Design review of the part built by this model. Coordinates are the model's own, in mm. Give positions to 0.01 mm unless a question says otherwise; leave off trailing zeros. Write each loop counter-clockwise with the first axis right and the second up, starting at its lowest first coordinate (ties: lowest second). Pieces come first, ordered by that corner, then holes. Notation, with made-up numbers: (8.5, -15.5) -> (28.5, -15.5) arc R20 cw to (28.5, 7.5) -> close; hole circle Ø6 at (72.25, 84.25). An arc over 180 degrees is marked (long way). Use CSV: the item, a comma, the result in double quotes.
```python
from build123d import *

# Parameters (mm, degrees)
SKETCH3_R              = 100
SKETCH3_R_2            = 80
BOSS_EXTRUDE1_DEPTH    = 3
SPLIT2_SURFACE_1_BACK  = 283.859
SPLIT2_SURFACE_1_DEPTH = 567.718
SPLIT2_SURFACE_2_BACK  = 283.859
SPLIT2_SURFACE_2_DEPTH = 567.718
BODY_DELETE1_DEPTH     = 3
SKETCH5_R              = 15
BOSS_EXTRUDE2_DEPTH    = 3
SKETCH6_R              = 3.21
CUT_EXTRUDE1_DEPTH     = 3
SPLIT3_SURFACE_3_BACK  = 209.781
SPLIT3_SURFACE_3_DEPTH = 419.562
SPLIT3_SURFACE_4_BACK  = 209.781
SPLIT3_SURFACE_4_DEPTH = 419.562
SPLIT4_SURFACE_5_BACK  = 209.781
SPLIT4_SURFACE_5_DEPTH = 419.562
SPLIT4_SURFACE_6_BACK  = 209.781
SPLIT4_SURFACE_6_DEPTH = 419.562
FILLET1_R              = 10
SPLIT5_SURFACE_7_BACK  = 207.768
SPLIT5_SURFACE_7_DEPTH = 415.536
SPLIT5_SURFACE_8_BACK  = 207.768
SPLIT5_SURFACE_8_DEPTH = 415.536


# Read off the part's stored shape, not the designer's step: Body-Delete1
with BuildPart() as part:
    # Sketch3 → Boss-Extrude1 (new body)
    with BuildSketch(Plane(origin=(0, 0, 0), x_dir=(1, 0, 0), z_dir=(0, 1, 0))):
        with Locations(Location((0, 0, 0), (0, 0, 270))):
            Circle(SKETCH3_R)
        with Locations(Location((0, 0, 0), (0, 0, 270))):
            Circle(SKETCH3_R_2, mode=Mode.SUBTRACT)
    extrude(amount=BOSS_EXTRUDE1_DEPTH)


with BuildPart() as body_2:
    # Split2: the piece behind the surface
    add(part.part)
    # Split2 surface: a surface, the sketch's curves swept straight by 567.718 mm
    with BuildLine(Plane(origin=(0, 3, 0), x_dir=(1, 0, 0), z_dir=(0, 1, 0)).offset(-SPLIT2_SURFACE_1_BACK), mode=Mode.PRIVATE) as split2_surface_1_path:
        Line((69.282032303, 72.111025509), (69.282032303, 40))
        Line((69.282032303, 40), (69.282032303, 0))
        Line((69.282032303, 0), (-114.167790304, 0))
        Line((-114.167790304, 0), (-114.167790304, -108.297460661))
        Line((-114.167790304, -108.297460661), (110.524137422, -108.297460661))
        Line((110.524137422, -108.297460661), (110.524137422, 72.111025509))
        Line((110.524137422, 72.111025509), (69.282032303, 72.111025509))
    split2_surface_1 = Shell.extrude(split2_surface_1_path.wire(), (0 * SPLIT2_SURFACE_1_DEPTH, 1 * SPLIT2_SURFACE_1_DEPTH, 0 * SPLIT2_SURFACE_1_DEPTH))
    split(bisect_by=split2_surface_1, keep=Keep.BOTTOM)

    # Sketch5 → Boss-Extrude2 (add)
    with BuildSketch(Plane(origin=(0, 3, 0), x_dir=(1, 0, 0), z_dir=(0, 1, 0))):
        with Locations((-89.945938306, 0)):
            Circle(SKETCH5_R)
    extrude(amount=-BOSS_EXTRUDE2_DEPTH)

    # Sketch6 → Cut-Extrude1 (cut)
    with BuildSketch(Plane(origin=(0, 3, 0), x_dir=(1, 0, 0), z_dir=(0, 1, 0))):
        with Locations(Location((-89.945938306, 0, 0), (0, 0, 270))):
            Circle(SKETCH6_R)
    extrude(amount=-CUT_EXTRUDE1_DEPTH, mode=Mode.SUBTRACT)


with BuildPart() as part_1:
    add(part.part)

    # Split2: split by a surface, the side it looks to stays
    # Split2 surface: a surface, the sketch's curves swept straight by 567.718 mm
    with BuildLine(Plane(origin=(0, 3, 0), x_dir=(1, 0, 0), z_dir=(0, 1, 0)).offset(-SPLIT2_SURFACE_2_BACK), mode=Mode.PRIVATE) as split2_surface_2_path:
        Line((69.282032303, 72.111025509), (69.282032303, 40))
        Line((69.282032303, 40), (69.282032303, 0))
        Line((69.282032303, 0), (-114.167790304, 0))
        Line((-114.167790304, 0), (-114.167790304, -108.297460661))
        Line((-114.167790304, -108.297460661), (110.524137422, -108.297460661))
        Line((110.524137422, -108.297460661), (110.524137422, 72.111025509))
        Line((110.524137422, 72.111025509), (69.282032303, 72.111025509))
    split2_surface_2 = Shell.extrude(split2_surface_2_path.wire(), (0 * SPLIT2_SURFACE_2_DEPTH, 1 * SPLIT2_SURFACE_2_DEPTH, 0 * SPLIT2_SURFACE_2_DEPTH))
    split(bisect_by=split2_surface_2, keep=Keep.TOP)

    # Body-Delete1 outline → Body-Delete1 (cut)
    with BuildSketch(Plane(origin=(0, 0, 0), x_dir=(1, 0, 0), z_dir=(0, 1, 0))):
        with BuildLine():
            ThreePointArc((-100, 0), (39.190539482, -92.000552255), (69.282032303, 72.111025509))
            Line((69.282032303, 72.111025509), (69.282032303, 40))
            ThreePointArc((69.282032303, 40), (20.705523608, -77.274066103), (-80, 0))
            Line((-80, 0), (-100, 0))
        make_face()
    extrude(amount=BODY_DELETE1_DEPTH, mode=Mode.SUBTRACT)


with BuildPart() as body_2_2:
    # Split3: the piece behind the surface
    add(body_2.part)
    # Split3 surface: a surface, the sketch's curves swept straight by 419.562 mm
    with BuildLine(Plane(origin=(0, 3, 0), x_dir=(1, 0, 0), z_dir=(0, 1, 0)).offset(-SPLIT3_SURFACE_3_BACK), mode=Mode.PRIVATE) as split3_surface_3_path:
        Line((69.282032303, 40), (59.018656665, 80.726688062))
        Line((59.018656665, 80.726688062), (73.479070656, 80.726688062))
        Line((73.479070656, 80.726688062), (69.282032303, 40))
    split3_surface_3 = Shell.extrude(split3_surface_3_path.wire(), (0 * SPLIT3_SURFACE_3_DEPTH, 1 * SPLIT3_SURFACE_3_DEPTH, 0 * SPLIT3_SURFACE_3_DEPTH))
    split(bisect_by=split3_surface_3, keep=Keep.BOTTOM)


with BuildPart() as body_2_1:
    add(body_2.part)

    # Split3: split by a surface, the side it looks to stays
    # Split3 surface: a surface, the sketch's curves swept straight by 419.562 mm
    with BuildLine(Plane(origin=(0, 3, 0), x_dir=(1, 0, 0), z_dir=(0, 1, 0)).offset(-SPLIT3_SURFACE_4_BACK), mode=Mode.PRIVATE) as split3_surface_4_path:
        Line((69.282032303, 40), (59.018656665, 80.726688062))
        Line((59.018656665, 80.726688062), (73.479070656, 80.726688062))
        Line((73.479070656, 80.726688062), (69.282032303, 40))
    split3_surface_4 = Shell.extrude(split3_surface_4_path.wire(), (0 * SPLIT3_SURFACE_4_DEPTH, 1 * SPLIT3_SURFACE_4_DEPTH, 0 * SPLIT3_SURFACE_4_DEPTH))
    split(bisect_by=split3_surface_4, keep=Keep.TOP)


with BuildPart() as body_2_3:
    # Split4: the piece behind the surface
    add(body_2_1.part)
    # Split4 surface: a surface, the sketch's curves swept straight by 419.562 mm
    with BuildLine(Plane(origin=(0, 3, 0), x_dir=(1, 0, 0), z_dir=(0, 1, 0)).offset(-SPLIT4_SURFACE_5_BACK), mode=Mode.PRIVATE) as split4_surface_5_path:
        Line((66.865251706, 49.590165356), (62.98651951, 48.612701009))
        Line((62.98651951, 48.612701009), (66.652010809, 34.067455273))
        Line((66.652010809, 34.067455273), (71.500426054, 35.289285706))
        Line((71.500426054, 35.289285706), (67.834934755, 49.834531442))
        Line((67.834934755, 49.834531442), (66.865251706, 49.590165356))
    split4_surface_5 = Shell.extrude(split4_surface_5_path.wire(), (0 * SPLIT4_SURFACE_5_DEPTH, 1 * SPLIT4_SURFACE_5_DEPTH, 0 * SPLIT4_SURFACE_5_DEPTH))
    split(bisect_by=split4_surface_5, keep=Keep.BOTTOM)

    # Fillet1
    # the kernel refuses this fillet: 10 mm, written as the material it takes off along each edge
    with BuildSketch(Plane(origin=(63.446918188, 16.684080126, -48.728724305), x_dir=(-0.6358841650465459, 0, -0.7717845092012777), z_dir=(0, -1, 0))) as fillet1_piece_1:
        with BuildLine():
            CenterArc((5.815734054, 9.994146598), FILLET1_R, 222.907386502, 45.132130872)
            Line((-1.508817296, 3.185993579), (-1.655308323, 3.049830519))
            ThreePointArc((-1.655308323, 3.049830519), (-0.935163624, 1.507395163), (-0.180754976, -0.085601627))
            Line((-0.180754976, -0.085601627), (0.00684204, -0.199882932))
            ThreePointArc((0.00684204, -0.199882932), (2.736816025, -0.153172783), (5.46679001, -0.199882932))
            Line((5.46679001, -0.199882932), (5.47363205, 0))
        make_face()
    extrude(amount=30.368160252, mode=Mode.SUBTRACT)


with BuildPart() as body_2_4:
    add(body_2_1.part)

    # Split4: split by a surface, the side it looks to stays
    # Split4 surface: a surface, the sketch's curves swept straight by 419.562 mm
    with BuildLine(Plane(origin=(0, 3, 0), x_dir=(1, 0, 0), z_dir=(0, 1, 0)).offset(-SPLIT4_SURFACE_6_BACK), mode=Mode.PRIVATE) as split4_surface_6_path:
        Line((66.865251706, 49.590165356), (62.98651951, 48.612701009))
        Line((62.98651951, 48.612701009), (66.652010809, 34.067455273))
        Line((66.652010809, 34.067455273), (71.500426054, 35.289285706))
        Line((71.500426054, 35.289285706), (67.834934755, 49.834531442))
        Line((67.834934755, 49.834531442), (66.865251706, 49.590165356))
    split4_surface_6 = Shell.extrude(split4_surface_6_path.wire(), (0 * SPLIT4_SURFACE_6_DEPTH, 1 * SPLIT4_SURFACE_6_DEPTH, 0 * SPLIT4_SURFACE_6_DEPTH))
    split(bisect_by=split4_surface_6, keep=Keep.TOP)


with BuildPart() as body_2_4_1:
    # Split5: the piece behind the surface
    add(body_2_3.part)
    # Split5 surface: a surface, the sketch's curves swept straight by 415.536 mm
    with BuildLine(Plane(origin=(0, 3, 0), x_dir=(1, 0, 0), z_dir=(0, 1, 0)).offset(-SPLIT5_SURFACE_7_BACK), mode=Mode.PRIVATE) as split5_surface_7_path:
        Line((60.973585358, 72.969223669), (58.06453621, 72.23612541))
        Line((58.06453621, 72.23612541), (60.508197077, 62.539294919))
        Line((60.508197077, 62.539294919), (68.981543377, 64.674630251))
        Line((68.981543377, 64.674630251), (66.537882511, 74.371460742))
        Line((66.537882511, 74.371460742), (60.973585358, 72.969223669))
    split5_surface_7 = Shell.extrude(split5_surface_7_path.wire(), (0 * SPLIT5_SURFACE_7_DEPTH, 1 * SPLIT5_SURFACE_7_DEPTH, 0 * SPLIT5_SURFACE_7_DEPTH))
    split(bisect_by=split5_surface_7, keep=Keep.BOTTOM)


with BuildPart() as body_2_3_1:
    add(body_2_3.part)

    # Split5: split by a surface, the side it looks to stays
    # Split5 surface: a surface, the sketch's curves swept straight by 415.536 mm
    with BuildLine(Plane(origin=(0, 3, 0), x_dir=(1, 0, 0), z_dir=(0, 1, 0)).offset(-SPLIT5_SURFACE_8_BACK), mode=Mode.PRIVATE) as split5_surface_8_path:
        Line((60.973585358, 72.969223669), (58.06453621, 72.23612541))
        Line((58.06453621, 72.23612541), (60.508197077, 62.539294919))
        Line((60.508197077, 62.539294919), (68.981543377, 64.674630251))
        Line((68.981543377, 64.674630251), (66.537882511, 74.371460742))
        Line((66.537882511, 74.371460742), (60.973585358, 72.969223669))
    split5_surface_8 = Shell.extrude(split5_surface_8_path.wire(), (0 * SPLIT5_SURFACE_8_DEPTH, 1 * SPLIT5_SURFACE_8_DEPTH, 0 * SPLIT5_SURFACE_8_DEPTH))
    split(bisect_by=split5_surface_8, keep=Keep.TOP)


solid = body_2_4_1.part
```
(1) For line 1 along X through (y, z) = (2.25, 0); line 2 along X through (y, z) = (2.65, -44.5); line 3 along X through (y, z) = (0.5, -63.5), list the stretches that pass through material, from the lowest coordinate up. Write a range as [from, to].
Established:
line 1,"x = [-104.95, -93.16], [-86.74, -74.95]"
line 2,"x = [-89.55, -66.48]"
line 3,"x = [-77.25, -48.66], [48.66, 60.27]"
(2) Mouldability with a two-part tool opening along Z and no side actions: class faces 1 (the face through (-45, 3, -68)), 2 (the face through (63.13, 1.52, -50.56)), 3 (the face through (-38.614, 1.479, -92.244)), 4 (the face through (-92.794, 1.521, 1.481)) as +Z half, -Z half, draft (parallel to the pull), parting line (faces both ways), or undercut.
Established:
face 1,"draft"
face 2,"+Z half"
face 3,"-Z half"
face 4,"undercut"
(3) Take a section at A-A (z = 0). Write out the cut boundary in (x, y).
Established:
outline,"(-104.95, 0) -> (-93.16, 0) -> (-93.16, 3) -> (-104.95, 3) -> close; (-86.74, 0) -> (-74.95, 0) -> (-74.95, 3) -> (-86.74, 3) -> close"
(4) Take a section at C-C (x = -71). Write out the cut boundary in (y, z), then the cut area to 3 significant figures.
Established:
outline,"(0, -70.42) -> (3, -70.42) -> (3, -36.86) -> (0, -36.86) -> close"
area,"101 mm2"
(5) Clearance check with flat-ended pins moving along their axes: pin 1 (1 mm diameter, centred on y = 2.5, z = 2.5, fed in from -X); pin 2 (6 mm diameter, centred on x = -89.95, z = 0, fed in from -Y); pin 3 (1.5 mm diameter, centred on x = 18.5, y = 2, fed in from +Z). State where each tip first meets the part, or that it passes through.
Established:
pin 1,"stops at x = -104.81"
pin 2,"passes through"
pin 3,"stops at z = -77.65"
(6) Take a section at B-B (y = 0.55). Write out the cut boundary in (x, z).
Established:
outline,"(-99.31, -11.72) arc R100 ccw to (59.02, -80.73) -> (60.97, -72.97) -> (58.06, -72.24) -> (60.51, -62.54) -> (63.42, -63.27) -> (66.87, -49.59) arc R10 ccw to (59.97, -52.95) arc R80 cw to (-79.3, -10.57) arc R15 ccw (long way) to start; hole circle Ø6.42 at (-89.95, 0)"
(7) Take a section at D-D (z = -25). Write out the cut boundary in (x, y).
Established:
outline,"(-96.82, 0) -> (-75.99, 0) -> (-75.99, 3) -> (-96.82, 3) -> close"
